The model under review builds one solid part; all positions refer to its coordinate system, in mm. A direction names the side the tool comes from. Give positions to 0.01 mm unless a question says otherwise; leave off trailing zeros. Order: outer loops, then holes, each group sorted by start corner. A loop starts at its lowest first (then second) coordinate and runs counter-clockwise, first axis right, second up. Notation, with made-up numbers: (78.5, 69) - (107.5, 69) arc R17 ccw to (107.5, 80) - close; hole circle Ø11 at (30.5, 54.25). An arc over 180 degrees is marked (long way). Use CSV: the item, a comma, the result in double quotes. Start each with the question number.
```python
from build123d import *

# Parameters (mm, degrees)
F0_R            = 12.7
F1_DEPTH        = 3.175
F2_R            = 0.3175
F4_DEPTH        = 6.351
F4_COPIES_COUNT = 10
F7_DEPTH        = 0.254


# Not quite as in the source:
# - a pattern or mirror of a feature is missing from the dataset's text; its kind, count and spacing are read off the source's solid


with BuildPart() as f1:
    # F0 (on Right) → F1 (new body, symmetric)
    with BuildSketch(Plane.YZ):
        Circle(F0_R)
    extrude(amount=F1_DEPTH, both=True)

    # F2 (on face) → F4 (cut, through all)
    with BuildSketch(Plane(origin=(-3.175, 0, 0), x_dir=(0, -1, 0), z_dir=(-1, 0, 0))):
        with Locations((0, 11.43)):
            Circle(F2_R)
    f4 = extrude(amount=-F4_DEPTH, mode=Mode.SUBTRACT)

    # F4_copies: F4 ×10 about axis
    f4_copies_axis = Axis((0, 0, 0), (1, 0, 0))
    for i in range(1, F4_COPIES_COUNT):
        add(f4.rotate(f4_copies_axis, i * 360 / F4_COPIES_COUNT), mode=Mode.SUBTRACT)

    # F5 (on face) → F7 (cut)
    with BuildSketch(Plane(origin=(-3.175, 0, 0), x_dir=(0, -1, 0), z_dir=(-1, 0, 0))):
        with BuildLine():
            ThreePointArc((-3.175, 0.254), (-3.429, 0), (-3.175, -0.254))
            Line((-3.175, -0.254), (0, -0.254))
            Line((0, -0.254), (3.175, -0.254))
            ThreePointArc((3.175, -0.254), (3.429, 0), (3.175, 0.254))
            Line((3.175, 0.254), (0, 0.254))
            Line((0, 0.254), (-3.175, 0.254))
        make_face()
    extrude(amount=-F7_DEPTH, mode=Mode.SUBTRACT)

    # F6 (on face) → F9 section 0
    with BuildSketch(Plane.YZ.offset(3.175)):
        with BuildLine():
            ThreePointArc((-3.175, 2.54), (-5.715, 0), (-3.175, -2.54))
            Line((-3.175, -2.54), (0, -2.54))
            Line((0, -2.54), (3.175, -2.54))
            ThreePointArc((3.175, -2.54), (5.715, 0), (3.175, 2.54))
            Line((3.175, 2.54), (0, 2.54))
            Line((0, 2.54), (-3.175, 2.54))
        make_face()
    # F8 (on face) → F9 section 1
    with BuildSketch(Plane(origin=(-2.921, 0, 0), x_dir=(0, -1, 0), z_dir=(-1, 0, 0))):
        with BuildLine():
            ThreePointArc((-3.175, 0.254), (-3.429, 0), (-3.175, -0.254))
            Line((-3.175, -0.254), (0, -0.254))
            Line((0, -0.254), (3.175, -0.254))
            ThreePointArc((3.175, -0.254), (3.429, 0), (3.175, 0.254))
            Line((3.175, 0.254), (0, 0.254))
            Line((0, 0.254), (-3.175, 0.254))
        make_face()
    loft(mode=Mode.SUBTRACT)


solid = f1.part
```
1. Consider section D-D (y = 2.75). Give the boundary of the cut face in (x, z) (3 decimals), and give its area (3 significant figures).
2. Consider section B-B (z = -11.43). Give the boundary of the cut face in (x, y) (1 decimal).
3. Clearance check with flat-ended pins moving along their axes: pin 1 (3 mm diameter, centred on x = -1.5, y = 2, fed in from +Z); pin 2 (3 mm diameter, centred on x = 2.5, y = -10, fed in from +Z). State where each tip first meets the part, or that it passes through.
4. Consider section A-A (y = 0). State how many separate pieces and enclosed holes the cut face has, and give its area (3 significant figures).
5. Tool access review of faces 1 (the face through (0.084, 4.556, -0.03)), 2 (the face through (3.175, 0, -3)): name each direction out of +Z, -Z, +X, -X, +Y, -Y from which nothing blocks a thin tool from reaching the whole face with its end or side.
6. Mouldability with a two-part tool opening along Y and no side actions: class faces 3 (the face through (0.08, 0.04, 1.38)), 4 (the face through (-3.175, 0, -3)), 5 (the face through (0.04, -2.75, -12.4)), 6 (the face through (0.084, -4.556, 0.03)) as pulls with the +Y half, pulls with the -Y half, needs draft (parallel to the pull), parting line crosses it, or undercut.
7. To check wall thickness, follow L1, parallel to Y at x = 1.75, z = 9.5; L2, parallel to Y at x = 1.25, z = 6; L3, parallel to Z at x = -1.5, y = 0. State the ranges of each line that lie inside material, in increasing order. Write a range as [from, to].
Answers follow:
1,outline,"(-3.175, -12.399) - (3.175, -12.399) - (3.175, -2.54) - (-2.921, -0.254) - (-3.175, -0.254) - close; (-3.175, 0.254) - (-2.921, 0.254) - (3.175, 2.54) - (3.175, 12.399) - (-3.175, 12.399) - close"
1,area,"140 mm^2"
2,outline,"(-3.2, -5.5) - (3.2, -5.5) - (3.2, -0.3) - (-3.2, -0.3) - close; (-3.2, 0.3) - (3.2, 0.3) - (3.2, 5.5) - (-3.2, 5.5) - close"
3,pin 1,"stops at z = 12.69"
3,pin 2,"stops at z = 9.44"
4,separate pieces,"4"
4,enclosed holes,"0"
4,area,"136 mm^2"
5,face 1,"+X"
5,face 2,"+Z, -Z, +X, +Y, -Y"
6,face 3,"undercut"
6,face 4,"needs draft"
6,face 5,"parting line crosses it"
6,face 6,"undercut"
7,L1,"y = [-8.43, -6.91], [-6.53, 6.53], [6.91, 8.43]"
7,L2,"y = [-11.19, 11.19]"
7,L3,"z = [-12.7, -11.75], [-11.11, -0.79], [0.79, 11.11], [11.75, 12.7]"
